```python
from build123d import *

# Parameters (mm, degrees)
SKETCH_1_R      = 1.525
EXTRUDE_1_DEPTH = 3
SKETCH_2_R      = 10
SKETCH_2_R_2    = 7
EXTRUDE_2_DEPTH = 5.1
CHAMFER_1_SIZE  = 2


with BuildPart() as part:
    # Эскиз1 → Бобышка-Вытянуть1 (new body)
    with BuildSketch(Plane.XY):
        with BuildLine():
            Line((13, 16), (-13, 16))
            ThreePointArc((-13, 16), (-15.121320344, 15.121320344), (-16, 13))
            Line((-16, 13), (-16, -13))
            ThreePointArc((-16, -13), (-15.121320344, -15.121320344), (-13, -16))
            Line((-13, -16), (13, -16))
            ThreePointArc((13, -16), (15.121320344, -15.121320344), (16, -13))
            Line((16, -13), (16, 13))
            ThreePointArc((16, 13), (15.121320344, 15.121320344), (13, 16))
        make_face()
        with Locations((-11.5, -11.5)):
            Circle(SKETCH_1_R, mode=Mode.SUBTRACT)
        with Locations((-11.5, 11.5)):
            Circle(SKETCH_1_R, mode=Mode.SUBTRACT)
        with Locations((11.5, -11.5)):
            Circle(SKETCH_1_R, mode=Mode.SUBTRACT)
        with Locations((11.5, 11.5)):
            Circle(SKETCH_1_R, mode=Mode.SUBTRACT)
    extrude(amount=EXTRUDE_1_DEPTH)

    # Эскиз2 → Бобышка-Вытянуть2 (add)
    with BuildSketch(Plane(origin=(0, 0, 0), x_dir=(-1, 0, 0), z_dir=(0, 0, -1))):
        with Locations(Location((0, 0, 0), (0, 0, 180))):
            Circle(SKETCH_2_R)
        Circle(SKETCH_2_R_2, mode=Mode.SUBTRACT)
    extrude(amount=EXTRUDE_2_DEPTH)

    # Фаска1
    chamfer_1_edges = [part.edges().sort_by_distance(p)[0] for p in [
        (-13.025, -11.5, 3),
        (9.975, -11.5, 3),
        (9.975, 11.5, 3),
        (-13.025, 11.5, 3),
    ]]
    chamfer(chamfer_1_edges, length=CHAMFER_1_SIZE)


solid = part.part
```
The model under review builds one solid part; all positions refer to its coordinate system, in mm. A direction names the side the tool comes from. Round coordinates to 2 decimals unless told otherwise and drop trailing zeros. Loops run counter-clockwise (first coordinate to the right, second up) from the corner with the lowest first, then second, coordinate; pieces in that order, holes last.
Item 1: For line 1 (Y direction, x = -11.5, z = 0.65) (3 decimals); line 2 (Y direction, x = 10.5, z = 2); line 3 (Z direction, x = 4, y = 4), list the stretches that pass through material, from the lowest coordinate up.
Determined:
line 1: y = -16 to -13.025, -9.975 to 9.975, 13.025 to 16
line 2: y = -16 to -13.82, -9.18 to 9.18, 13.82 to 16
line 3: z = 0 to 3
Item 2: Clearance check with flat-ended pins moving along their axes: pin 1 Ø3.5 at (x, y) = (11.5, -11.5) entering from +Z (3 decimals); pin 2 Ø1.5 at (y, z) = (9.5, -3.5) entering from -X; pin 3 Ø1.5 at (x, y) = (-3, -3) entering from -Z. State where each tip first meets the part, or that it passes through.
Determined:
pin 1: stops at z = 1.225
pin 2: stops at x = -4.84
pin 3: stops at z = 0
Item 3: For faces 4 (the face through (-6.466, -2.681, -2.514)), 5 (the face through (-10.1, 10.9, 0.5)), list the 3-axis set-ups (+Z, -Z, +X, -X, +Y, -Y) from which the entire face can be reached by the end or side of a thin tool; tool diameter is ignored.
Determined:
face 4: -Z
face 5: +Z, -Z
Item 4: Take a section at D-D (z = -3.25). Write out the cut boundary in (x, y).
Determined:
outline: circle Ø20 at (0, 0); hole circle Ø14 at (0, 0)
Item 5: Mouldability with a two-part tool opening along Y and no side actions: class faces 1 (the face through (15.14, 15.1, 1.48)), 2 (the face through (12.955, -11.042, 0.493)), 3 (the face through (-7.3, 7.3, 0)) as released by +Y, released by -Y, zero draft, split by the parting line, or undercut.
Determined:
face 1: released by +Y
face 2: undercut
face 3: zero draft
Item 6: Take a section at C-C (y = 0). Write out the cut boundary in (x, z), then the cut area to 3 significant figures.
Determined:
outline: (-16, 0) - (-10, 0) - (-10, -5.1) - (-7, -5.1) - (-7, 0) - (7, 0) - (7, -5.1) - (10, -5.1) - (10, 0) - (16, 0) - (16, 3) - (-16, 3) - close
area: 127 mm2
Item 7: Take a section at A-A (x = 11.5). Write out the cut boundary in (y, z) (3 decimals).
Determined:
outline: (-16, 0) - (-13.025, 0) - (-13.025, 1) - (-15.025, 3) - (-16, 3) - close; (-9.975, 0) - (9.975, 0) - (9.975, 1) - (7.975, 3) - (-7.975, 3) - (-9.975, 1) - close; (13.025, 0) - (16, 0) - (16, 3) - (15.025, 3) - (13.025, 1) - close
